from build123d import *

# Parameters (mm, degrees)
SKETCH1_W           = 130
SKETCH1_H           = 40
BOSS_EXTRUDE1_DEPTH = 2
SKETCH2_W           = 40
SKETCH2_H           = 35
BOSS_EXTRUDE2_DEPTH = 2


with BuildPart() as part:
    # Sketch1 → Boss-Extrude1 (new body)
    with BuildSketch(Plane(origin=(0, 0, 0), x_dir=(1, 0, 0), z_dir=(0, 1, 0))):
        with Locations((65, 20)):
            Rectangle(SKETCH1_W, SKETCH1_H)
    extrude(amount=BOSS_EXTRUDE1_DEPTH)

    # Sketch2 → Boss-Extrude2 (add)
    with BuildSketch(Plane.ZY):
        with Locations((-20, -15.5)):
            Rectangle(SKETCH2_W, SKETCH2_H)
    boss_extrude2 = extrude(amount=-BOSS_EXTRUDE2_DEPTH)

    # Mirror1: Boss-Extrude2 across plane
    add(boss_extrude2.mirror(Plane(origin=(65, 0, 0), x_dir=(0, 0, 1), z_dir=(1, 0, 0))))


solid = part.part
Source: CAD feature listing. Evaluate the final solid. Frame: model axes, mm. A direction names the side the tool comes from. Give positions to 0.01 mm unless a question says otherwise; leave off trailing zeros. Loops run counter-clockwise (first coordinate to the right, second up) from the corner with the lowest first, then second, coordinate; pieces in that order, holes last. Notation, with made-up numbers: (37.5, 86) -> (90.5, 86) arc R18 cw to (90.5, 115) -> close; hole circle Ø4 at (-25.75, -13). An arc over 180 degrees is marked (long way). Use a Markdown table: item, result. Add a question column.
1) Pull-direction query (X, two-part tool) for faces 1 (the face through (0, -15, -20)), 2 (the face through (2, -16, -20)), 3 (the face through (65, 1, -40)); classes: +X half, -X half, draft (parallel to the pull), parting line (faces both ways), or undercut.
2) Line query: line 1 along X through (y, z) = (-13.5, -5.5); line 2 along Y through (x, z) = (93, -25). Output: solid intervals per line, ascending. Write a range as [from, to].
3) Reachability of faces 4 (the face through (64, 0, -20)), 5 (the face through (64, 2, -20)) from +Z, -Z, +X, -X, +Y, -Y: full face, straight path, thin tool, end or side. Return the list, or none.
4) Section query A-A, the plane y = -29. Return the cut outline in (x, z), then the cut area to 3 significant figures.
5) Section query C-C, the plane x = 66. Return the cut outline in (y, z).
6) First-contact query: pin 1 (12 mm diameter, centred on x = 20, z = -32, fed in from -Y). Flat tip, straight axial feed; report the tip coordinate or a pass-through.
7) Section query B-B, the plane z = -2.5. Return the cut outline in (x, y).
Numbers:
| question | item | result |
|---|---|---|
| 1 | face 1 | -X half |
| 1 | face 2 | undercut |
| 1 | face 3 | draft |
| 2 | line 1 | x = [0, 2], [128, 130] |
| 2 | line 2 | y = [0, 2] |
| 3 | face 4 | +Z, -Z, -Y |
| 3 | face 5 | +Z, -Z, +X, -X, +Y |
| 4 | outline | (0, -40) -> (2, -40) -> (2, 0) -> (0, 0) -> close; (128, -40) -> (130, -40) -> (130, 0) -> (128, 0) -> close |
| 4 | area | 160 mm2 |
| 5 | outline | (0, -40) -> (2, -40) -> (2, 0) -> (0, 0) -> close |
| 6 | pin 1 | stops at y = 0 |
| 7 | outline | (0, -33) -> (2, -33) -> (2, 0) -> (128, 0) -> (128, -33) -> (130, -33) -> (130, 2) -> (0, 2) -> close |
